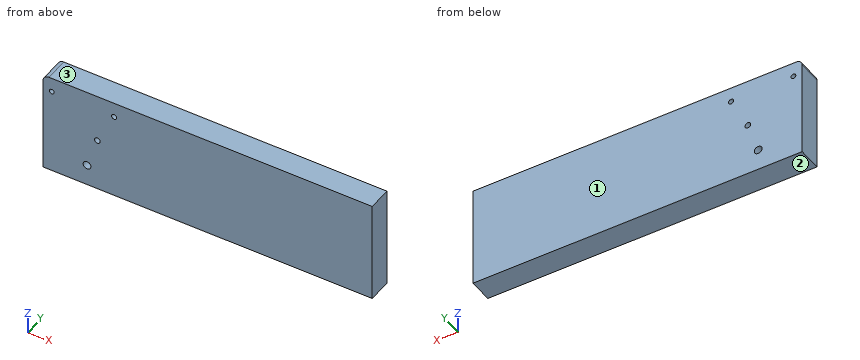
```python
from build123d import *

# Parameters (mm, degrees)
F0_R     = 4.145299883
F0_R_2   = 2.5851912666
F0_R_3   = 3.0648919033
F0_R_4   = 2.7118286766
F1_DEPTH = 25.4
F2_DEPTH = 254


# Not quite as in the source:
# - the program builds the solid bodies; features that only make, move or delete a surface that nothing else refers to are left out


with BuildPart() as f1:
    # F0 (on Front) → F1 (new body)
    with BuildSketch(Plane.XZ):
        with BuildLine():
            Line((50.6008081138, 51.9382767379), (-40.6842338085, 51.9382767379))
            ThreePointArc((-40.6842338085, 51.9382767379), (-45.1743618691, 50.0784047985), (-47.0342338085, 45.5882767379))
            Line((-47.0342338085, 45.5882767379), (-47.0342338085, -56.842315942))
            Line((-47.0342338085, -56.842315942), (50.6008081138, -56.842315942))
            Line((50.6008081138, -56.842315942), (50.6008081138, 51.9382767379))
        make_face()
        with Locations((0, -34.0232253075)):
            Circle(F0_R, mode=Mode.SUBTRACT)
        with Locations((-37.6131273806, 36.3515801728)):
            Circle(F0_R_2, mode=Mode.SUBTRACT)
        with Locations((10.9797539189, 0)):
            Circle(F0_R_3, mode=Mode.SUBTRACT)
        with Locations((28.9033185691, 35.878714174)):
            Circle(F0_R_4, mode=Mode.SUBTRACT)
    extrude(amount=F1_DEPTH)

    # F2 (add): a face of the model
    f2_faces = [f1.faces().sort_by_distance(p)[0] for p in [
        (50.6008081138, -12.7, -2.4520196021),
    ]]
    extrude(f2_faces, amount=F2_DEPTH)


solid = f1.part
```
Design review of the part built by this model. Coordinates are the model's own, in mm. Face numbers are marked on the shaded views. Round coordinates to 2 decimals unless told otherwise and drop trailing zeros. Order: outer loops, then holes, each group sorted by start corner. A loop starts at its lowest first (then second) coordinate and runs counter-clockwise, first axis right, second up. Notation, with made-up numbers: M 86,60.5 L 108,60.5 A26 ccw 108,85.5 Z; hole C -12,-2 d7. An arc over 180 degrees is marked long. Put each result on its own line as item: value.
Q1. To check wall thickness, follow line 1 (X direction, y = -19.75, z = 36); line 2 (X direction, y = -4, z = 37.5); line 3 (X direction, y = -11, z = -2). State the ranges of each line that lie inside material, in increasing order.
Reported:
line 1: -47.03 to -40.17, -35.05 to 26.19, 31.61 to 304.6
line 2: -47.03 to -39.93, -35.3 to 26.73, 31.08 to 304.6
line 3: -47.03 to 8.66, 13.3 to 304.6
Q2. Consider section A-A (z = 0). State the section outline as (x, y) points, and give its area (3 significant figures).
Reported:
outline: M -47.03,-25.4 L 7.91,-25.4 L 7.91,0 L -47.03,0 Z; M 14.04,-25.4 L 304.6,-25.4 L 304.6,0 L 14.04,0 Z
area: 8,780 mm²
Q3. Draft analysis for pull direction Z (two halves, no side actions). For the marked faces 1, 2 and 3, state which applies: released by +Z, released by -Z, zero draft, split by the parting line, or undercut.
Reported:
face 1: zero draft
face 2: released by -Z
face 3: released by +Z
Q4. Insertion check: pin 1 Ø5 at (x, z) = (10.98, 0) entering from -Y. The pin has a flat end and moves straight along its axis. Give the tip position at first contact, or say it passes through.
Reported:
pin 1: through
Q5. Consider section B-B (x = 0). State the section outline as (y, z) points.
Reported:
outline: M -25.4,-56.84 L 0,-56.84 L 0,-38.17 L -25.4,-38.17 Z; M -25.4,-29.88 L 0,-29.88 L 0,51.94 L -25.4,51.94 Z
